The figure shows three views and two pictorial views of one solid part (mm, origin at its lowest corner). Answer the questions. Give positions to 0.01 mm unless a question says otherwise; leave off trailing zeros. Loops run counter-clockwise (first coordinate to the right, second up) from the corner with the lowest first, then second, coordinate; pieces in that order, holes last. Notation, with made-up numbers: (36.25, 16.25) -> (43.25, 16.25) arc R8 cw to (43.25, 31.25) -> close; hole circle Ø6 at (-3, 1.25). An arc over 180 degrees is marked (long way). One line per item, written item: value. Start each with the question number.
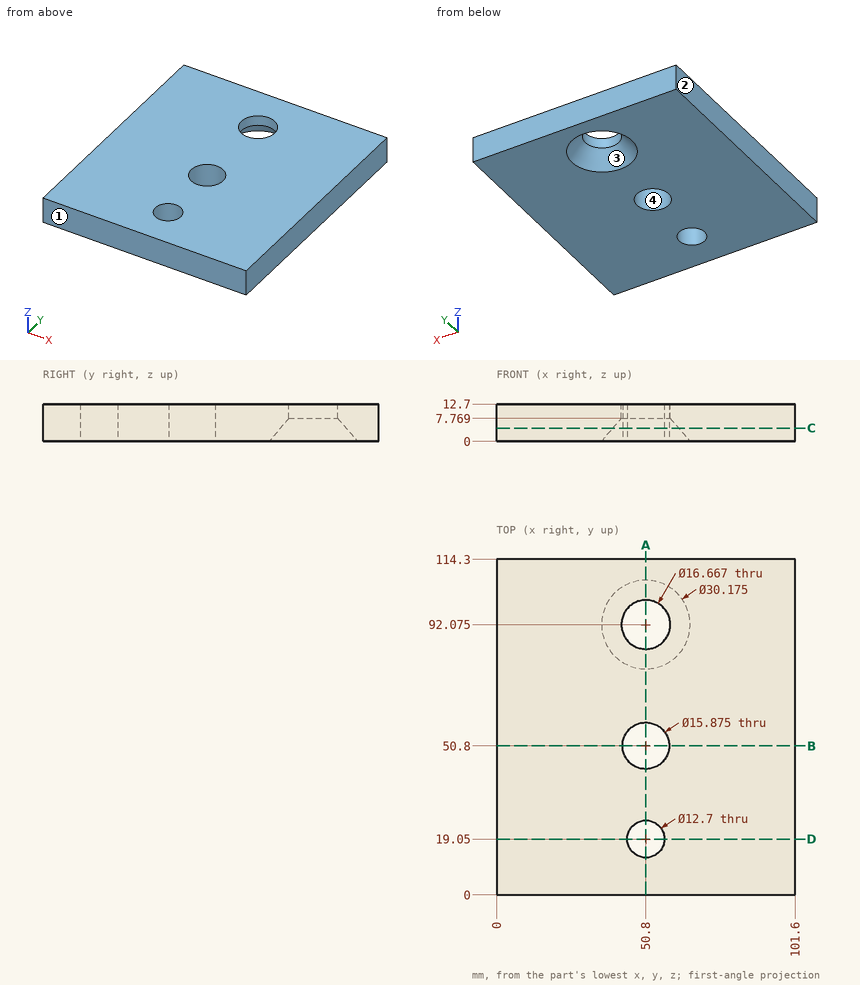
Item 1: Section B-B, the plane y = 50.8 is taken. Determine the outline of the cut face in (x, z).
Item 2: Section D-D, the plane y = 19.05 is taken. Determine the outline of the cut face in (x, z).
Item 3: Determine the mould class of the marked faces 1, 2, 3 and 4 for opening direction X: pulls with the +X half, pulls with the -X half, needs draft (parallel to the pull), parting line crosses it, or undercut.
Item 4: Section A-A, the plane x = 50.8 is taken. Determine the outline of the cut face in (y, z).
Item 5: Consider L1, parallel to Y at x = 50.8, z = 9; L2, parallel to Y at x = 50.8, z = 5 (1 decimal); L3, parallel to X at y = 15, z = 6.75. Determine where each line is inside the solid, lowest interval first. Write a range as [from, to].
Item 6: Section C-C, the plane z = 4.5 is taken. State how many separate pieces and enclosed holes the cut face has, plus the area to 3 significant figures.
Computed values:
1. outline: (0, 0) -> (42.86, 0) -> (42.86, 12.7) -> (0, 12.7) -> close; (58.74, 0) -> (101.6, 0) -> (101.6, 12.7) -> (58.74, 12.7) -> close
2. outline: (0, 0) -> (44.45, 0) -> (44.45, 12.7) -> (0, 12.7) -> close; (57.15, 0) -> (101.6, 0) -> (101.6, 12.7) -> (57.15, 12.7) -> close
3. face 1: needs draft
3. face 2: pulls with the -X half
3. face 3: undercut
3. face 4: undercut
4. outline: (0, 0) -> (12.7, 0) -> (12.7, 12.7) -> (0, 12.7) -> close; (25.4, 0) -> (42.86, 0) -> (42.86, 12.7) -> (25.4, 12.7) -> close; (58.74, 0) -> (76.99, 0) -> (83.74, 7.77) -> (83.74, 12.7) -> (58.74, 12.7) -> close; (100.41, 7.77) -> (107.16, 0) -> (114.3, 0) -> (114.3, 12.7) -> (100.41, 12.7) -> close
5. L1: [0, 12.7], [25.4, 42.86], [58.74, 83.74], [100.41, 114.3]
5. L2: [0, 12.7], [25.4, 42.9], [58.7, 81.3], [102.8, 114.3]
5. L3: [0, 45.91], [55.69, 101.6]
6. separate pieces: 1
6. enclosed holes: 3
6. area: 10,900 mm²
